Input: part model. Units: mm. Frame: model coordinates. Face numbers are marked on the shaded views. A direction names the side the tool comes from. Give positions to 0.01 mm unless a question says otherwise; leave off trailing zeros. Order: outer loops, then holes, each group sorted by start corner. A loop starts at its lowest first (then second) coordinate and runs counter-clockwise, first axis right, second up. Notation, with made-up numbers: (-23, 30) - (3, 30) arc R19 ccw to (3, 41) - close; hole circle Ø8 at (61.25, -23.75). An arc over 180 degrees is marked (long way). Answer in a Markdown table with one row per item. Add a question column.
from build123d import *

# Parameters (mm, degrees)
F0_W     = 45.25
F0_H     = 10
F1_DEPTH = 2
F2_W     = 45.25
F2_H     = 2
F3_DEPTH = 7
F4_R     = 0.5
F5_DEPTH = 25
F6_DEPTH = 25
F7_W     = 2.616208
F7_H     = 1.183311
F8_DEPTH = 3


with BuildPart() as f1:
    # F0 (on Top) → F1 (new body)
    with BuildSketch(Plane.XY):
        with Locations((22.625, 5)):
            Rectangle(F0_W, F0_H)
    extrude(amount=F1_DEPTH)

    # F2 (on face) → F3 (join)
    with BuildSketch(Plane.XY.offset(2)):
        with Locations((22.625, 1)):
            Rectangle(F2_W, F2_H)
    extrude(amount=F3_DEPTH)

    # F4 (on face) → F5 (cut)
    with BuildSketch(Plane.XZ):
        with Locations((2.975, 4.5)):
            Circle(F4_R)
    extrude(amount=-F5_DEPTH, mode=Mode.SUBTRACT)

    # F4 (on face) → F6 (cut)
    with BuildSketch(Plane.XZ):
        with Locations((42.275, 4.5)):
            Circle(F4_R)
    extrude(amount=-F6_DEPTH, mode=Mode.SUBTRACT)

    # F7 (on face) → F8 (cut)
    with BuildSketch(Plane.XY.offset(2)):
        with Locations((30.246938, 2.591655)):
            Rectangle(F7_W, F7_H)
    extrude(amount=-F8_DEPTH, mode=Mode.SUBTRACT)


solid = f1.part
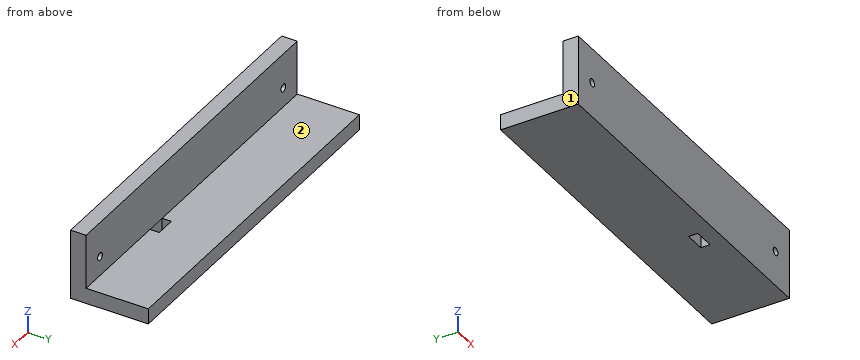
Q1. Access query for the marked faces 1 and 2. Directions: +Z, -Z, +X, -X, +Y, -Y. A direction counts if a zero-diameter tool reaches every point of the face in a straight line with its end or side. Return the directions, or none.
Q2. Line query: probe 1 along Y at (x, z) = (35.5, 7); probe 2 along X at (y, z) = (3, 1.5). Output: solid intervals per line, ascending.
Q3. Contact query for flat-ended pins moving along their axis: P1, Ø2.5, axis at x = 14, y = 7, coming from the +Z side; P2, Ø1, axis at x = 7, z = 7, coming from the +Y side. Output: stop coordinate, or through.
Q4. Section C-C, the plane y = 4. Return loops of the section in (x, z).
Q5. Section B-B, the plane x = 8. Return loops of the section in (y, z).
Q6. Section A-A, the plane z = 4.5. Return loops of the section in (x, y) (3 decimals), then the cut area to 3 significant figures.
Computed:
| question | item | result |
|---|---|---|
| 1 | face 1 | +Z, -Z, -X, +Y, -Y |
| 1 | face 2 | +Z, +X, -X, +Y |
| 2 | probe 1 | y = 0 to 2 |
| 2 | probe 2 | x = 0 to 28.94, 31.56 to 45.25 |
| 3 | P1 | stops at z = 2 |
| 3 | P2 | stops at y = 2 |
| 4 | outline | (0, 0) - (45.25, 0) - (45.25, 2) - (0, 2) - close |
| 5 | outline | (0, 0) - (10, 0) - (10, 2) - (2, 2) - (2, 9) - (0, 9) - close |
| 6 | outline | (0, 0) - (2.475, 0) - (2.475, 2) - (0, 2) - close; (3.475, 0) - (41.775, 0) - (41.775, 2) - (3.475, 2) - close; (42.775, 0) - (45.25, 0) - (45.25, 2) - (42.775, 2) - close |
| 6 | area | 86.5 mm^2 |
